Here's how the part is built. I have some questions about the finished solid (model axes, mm). Face numbers are marked on the shaded views. A direction names the side the tool comes from. Coordinates: 2 decimals unless noted, no trailing zeros. Order: outer loops, then holes, each group sorted by start corner. A loop starts at its lowest first (then second) coordinate and runs counter-clockwise, first axis right, second up. Notation, with made-up numbers: M -1,-25 L 22,-25 A20 ccw 22,-4 Z; hole C 22,46.25 d7. An arc over 180 degrees is marked long. One line per question, with ' | ' between items. Start each with the question number.
```python
from build123d import *

# Parameters (mm, degrees)
BOSS_EXTRUDE1_DEPTH = 10
FILLET1_R           = 1
SKETCH4_R           = 2.5
CUT_EXTRUDE1_DEPTH  = 11
FILLET2_R           = 0.5


with BuildPart() as part:
    # Sketch3 → Boss-Extrude1 (new body)
    with BuildSketch(Plane(origin=(0, 0, 0), x_dir=(1, 0, 0), z_dir=(0, 1, 0))):
        with BuildLine():
            Line((11, 27.75), (11, 29.5))
            ThreePointArc((11, 29.5), (10.646446609, 29.646446609), (10.5, 30))
            Line((10.5, 30), (0, 30))
            Line((0, 30), (0, 19.5))
            ThreePointArc((0, 19.5), (0.353553391, 19.353553391), (0.5, 19))
            Line((0.5, 19), (2.25, 19))
            Line((2.25, 19), (2.25, 22))
            Line((2.25, 22), (4.5, 22))
            Line((4.5, 22), (8.25, 18.5))
            Line((8.25, 18.5), (8.25, 15.5))
            Line((8.25, 15.5), (8.75, 15))
            Line((8.75, 15), (8.25, 14.5))
            Line((8.25, 14.5), (8.25, 11.5))
            Line((8.25, 11.5), (4.5, 8))
            Line((4.5, 8), (2.25, 8))
            Line((2.25, 8), (2.25, 11))
            Line((2.25, 11), (0.5, 11))
            ThreePointArc((0.5, 11), (0.353553391, 10.646446609), (0, 10.5))
            Line((0, 10.5), (0, 0))
            Line((0, 0), (10.5, 0))
            ThreePointArc((10.5, 0), (10.646446609, 0.353553391), (11, 0.5))
            Line((11, 0.5), (11, 2.25))
            Line((11, 2.25), (8, 2.25))
            Line((8, 2.25), (8, 4.5))
            Line((8, 4.5), (11.5, 8.25))
            Line((11.5, 8.25), (14.5, 8.25))
            Line((14.5, 8.25), (15, 8.75))
            Line((15, 8.75), (15.5, 8.25))
            Line((15.5, 8.25), (18.5, 8.25))
            Line((18.5, 8.25), (22, 4.5))
            Line((22, 4.5), (22, 2.25))
            Line((22, 2.25), (19, 2.25))
            Line((19, 2.25), (19, 0.5))
            ThreePointArc((19, 0.5), (19.353553391, 0.353553391), (19.5, 0))
            Line((19.5, 0), (30, 0))
            Line((30, 0), (30, 10.5))
            ThreePointArc((30, 10.5), (29.646446609, 10.646446609), (29.5, 11))
            Line((29.5, 11), (27.75, 11))
            Line((27.75, 11), (27.75, 8))
            Line((27.75, 8), (25.5, 8))
            Line((25.5, 8), (21.75, 11.5))
            Line((21.75, 11.5), (21.75, 14.5))
            Line((21.75, 14.5), (21.25, 15))
            Line((21.25, 15), (21.75, 15.5))
            Line((21.75, 15.5), (21.75, 18.5))
            Line((21.75, 18.5), (25.5, 22))
            Line((25.5, 22), (27.75, 22))
            Line((27.75, 22), (27.75, 19))
            Line((27.75, 19), (29.5, 19))
            ThreePointArc((29.5, 19), (29.646446609, 19.353553391), (30, 19.5))
            Line((30, 19.5), (30, 30))
            Line((30, 30), (19.5, 30))
            ThreePointArc((19.5, 30), (19.353553391, 29.646446609), (19, 29.5))
            Line((19, 29.5), (19, 27.75))
            Line((19, 27.75), (22, 27.75))
            Line((22, 27.75), (22, 25.5))
            Line((22, 25.5), (18.5, 21.75))
            Line((18.5, 21.75), (15.5, 21.75))
            Line((15.5, 21.75), (15, 21.25))
            Line((15, 21.25), (14.5, 21.75))
            Line((14.5, 21.75), (11.5, 21.75))
            Line((11.5, 21.75), (8, 25.5))
            Line((8, 25.5), (8, 27.75))
            Line((8, 27.75), (11, 27.75))
        make_face()
    extrude(amount=BOSS_EXTRUDE1_DEPTH)

    # Fillet1
    fillet1_edges = [part.edges().sort_by_distance(p)[0] for p in [
        (30, 5, 0),
        (0, 5, 0),
        (0, 5, -30),
        (30, 5, -30),
    ]]
    fillet(fillet1_edges, radius=FILLET1_R)

    # Sketch4 → Cut-Extrude1 (cut, through all)
    with BuildSketch(Plane(origin=(0, 10, 0), x_dir=(1, 0, 0), z_dir=(0, 1, 0))):
        with Locations((15, 15)):
            Circle(SKETCH4_R)
    extrude(amount=-CUT_EXTRUDE1_DEPTH, mode=Mode.SUBTRACT)

    # Fillet2
    fillet2_edges = [part.edges().sort_by_distance(p)[0] for p in [
        (27.75, 5, -19),
        (27.75, 5, -22),
        (21.75, 5, -15.5),
        (21.75, 5, -14.5),
        (27.75, 5, -8),
        (27.75, 5, -11),
        (19, 5, -2.25),
        (22, 5, -2.25),
        (15.5, 5, -8.25),
        (14.5, 5, -8.25),
        (8, 5, -2.25),
        (11, 5, -2.25),
        (2.25, 5, -11),
        (2.25, 5, -8),
        (8.25, 5, -14.5),
        (8.25, 5, -15.5),
        (2.25, 5, -22),
        (2.25, 5, -19),
        (11, 5, -27.75),
        (8, 5, -27.75),
        (14.5, 5, -21.75),
        (15.5, 5, -21.75),
        (22, 5, -27.75),
        (19, 5, -27.75),
    ]]
    fillet(fillet2_edges, radius=FILLET2_R)


solid = part.part
```
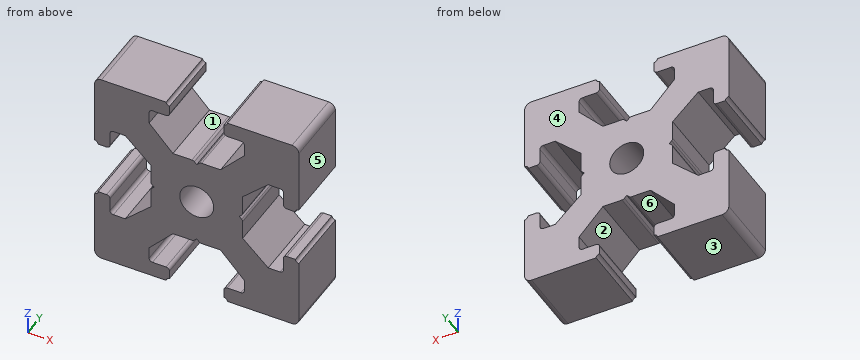
1. We'd pull the mould along X, two halves only. Please class the marked faces 4, 5 and 6: released by +X, released by -X, zero draft, split by the parting line, or undercut.
2. Imagine slicing it at C-C (x = 9.5). List the corners of the cut face in (y, z) for me.
3. Imagine slicing it at B-B (x = 26). List the corners of the cut face in (y, z) for me.
4. Imagine slicing it at A-A (z = -3.5). List the corners of the cut face in (x, y) for me, then the cut area to 3 significant figures.
5. I need wall thicknesses on line 1 (Z direction, x = 9.25, y = 8.75); line 2 (X direction, y = 4.5, z = -27); line 3 (X direction, y = 6.5, z = -20.5). Which ranges of each line are inside material? Lowest first, please.
6. Which directions (+Z, -Z, +X, -X, +Y, -Y) give clear straight access to the entire face, cutting with the end or side of a thin tool? Please do the marked faces 1, 2 and 3.
7. Will this pin go through, and if not, where does the flat tip stop? pin 1 (1.4 mm diameter, centred on x = 17.5, y = 5.5, fed in from -Z).
Entries:
1) face 4: zero draft | face 5: released by +X | face 6: undercut
2) outline: M 0,-30 L 10,-30 L 10,-27.75 L 0,-27.75 Z; M 0,-23.89 L 10,-23.89 L 10,-6.11 L 0,-6.11 Z; M 0,-2.25 L 10,-2.25 L 10,0 L 0,0 Z
3) outline: M 0,-30 L 10,-30 L 10,-22 L 0,-22 Z; M 0,-8 L 10,-8 L 10,0 L 0,0 Z
4) outline: M 0,0 L 8,0 L 8,10 L 0,10 Z; M 22,0 L 30,0 L 30,10 L 22,10 Z | area: 160 mm²
5) line 1: -30 to -27.75, -24.16 to -5.84, -2.25 to 0 | line 2: 0 to 8, 22 to 30 | line 3: 0 to 2.25, 6.11 to 23.89, 27.75 to 30
6) face 1: +Z, +Y, -Y | face 2: +Y, -Y | face 3: -Z, +X, -X, +Y, -Y
7) pin 1: z = -21.75
